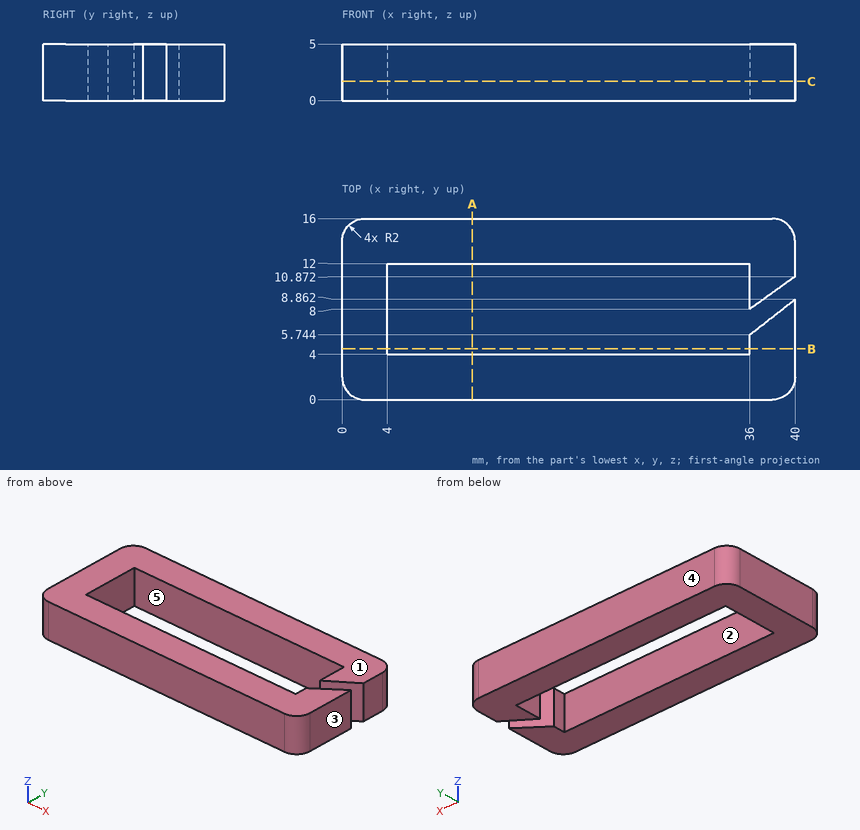
Geometry check sheet. Reference: drawing and pictorial views, mm from the part's lowest x, y, z. A direction names the side the tool comes from. Round coordinates to 2 decimals unless told otherwise and drop trailing zeros. Loops run counter-clockwise (first coordinate to the right, second up) from the corner with the lowest first, then second, coordinate; pieces in that order, holes last. Notation, with made-up numbers: (24.25, 89.5) - (72.25, 89.5) arc R22 cw to (72.25, 126.5) - close; hole circle Ø10 at (38, -8.5). An arc over 180 degrees is marked (long way). Use a Markdown table: item, result. Add a question column.
1. Release check for a two-part mould opening along Y. For the marked faces 3, 4 and 5 record: released by +Y, released by -Y, zero draft, split by the parting line, or undercut.
2. Thickness scan on probe 1 along Y at (x, z) = (5, 2.3); probe 2 along X at (y, z) = (11.5, 3.7); probe 3 along X at (y, z) = (10.25, 4.6) (1 decimal). Record the ranges inside material, lowest first. Write a range as [from, to].
3. Gauge pin test, flat end, axial feed: pin 1 (1.5 mm diameter, centred on x = 29.5, y = 10.5, fed in from -Z). Record the tip position at first contact, or that the pin passes through.
4. Section check A-A, the plane x = 11.5. Record the boundary of the cut face in (y, z).
5. Section check B-B, the plane y = 4.5. Record the boundary of the cut face in (x, z), plus the area to 3 significant figures.
6. Access from +Z, -Z, +X, -X, +Y, -Y to the whole of each face (thin tool, end or side, straight path). Record for the marked faces 1 and 2.
7. Section check C-C, the plane z = 1.7. Record the boundary of the cut face in (x, y).
Checks:
| question | item | result |
|---|---|---|
| 1 | face 3 | zero draft |
| 1 | face 4 | released by +Y |
| 1 | face 5 | undercut |
| 2 | probe 1 | y = [0, 4], [12, 16] |
| 2 | probe 2 | x = [0, 4], [36, 40] |
| 2 | probe 3 | x = [0, 4], [36, 39.1] |
| 3 | pin 1 | passes through |
| 4 | outline | (0, 0) - (4, 0) - (4, 5) - (0, 5) - close; (12, 0) - (16, 0) - (16, 5) - (12, 5) - close |
| 5 | outline | (0, 0) - (4, 0) - (4, 5) - (0, 5) - close; (36, 0) - (40, 0) - (40, 5) - (36, 5) - close |
| 5 | area | 40.0 mm^2 |
| 6 | face 1 | +Z, +X, -X, +Y, -Y |
| 6 | face 2 | +Z, -Z |
| 7 | outline | (0, 2) arc R2 ccw to (2, 0) - (38, 0) arc R2 ccw to (40, 2) - (40, 8.86) - (36, 5.74) - (36, 4) - (4, 4) - (4, 12) - (36, 12) - (36, 8) - (40, 10.87) - (40, 14) arc R2 ccw to (38, 16) - (2, 16) arc R2 ccw to (0, 14) - close |
